Could you check a few things on this model? Use its own coordinates, in mm. A direction names the side the tool comes from. Give positions to 0.01 mm unless a question says otherwise; leave off trailing zeros. Loops run counter-clockwise (first coordinate to the right, second up) from the corner with the lowest first, then second, coordinate; pieces in that order, holes last. Notation, with made-up numbers: M 58.5,66.5 L 100.5,66.5 A11 ccw 100.5,78.5 Z; hole C 2,14.5 d7. An arc over 180 degrees is marked long. Use a Markdown table: item, result. Add a question column.
1) Suppose I cut it at D-D on z = 1.75. List the corners of the cut face in (x, y) for me, and give its area (3 significant figures).
2) Suppose I cut it at A-A on z = 6. List the corners of the cut face in (x, y) for me, and give its area (3 significant figures).
3) If I drill on line 1 along X through (y, z) = (3.45, 6); line 2 along X through (y, z) = (1.8, 6); line 3 along Z through (x, y) = (-20, 4), over which ranges is the centre line in solid material (lowest first)? Write a range as [from, to].
4) Which directions (+Z, -Z, +X, -X, +Y, -Y) give clear straight access to the entire face, cutting with the end or side of a thin tool? Please do faces 5 (the flat face through (25, 15, 1)), 6 (the flat face through (-23.487, 17.602, 0.493)), 7 (the flat face through (21.1, 5, 6)), 8 (the flat face through (-30.92, 17.91, 0.49)).
5) We'd pull the mould along X, two halves only. Please class faces 1 (the flat face through (-25, 15, 1)), 2 (the flat face through (-27.14, 11.63, 0.49)), 3 (the flat face through (30.97, 17.82, 0.49)), 4 (the flat face through (23.64, 17.69, 0.49)): +X half, -X half, draft (parallel to the pull), parting line (faces both ways), or undercut.
6) Suppose I cut it at B-B on y = 12. List the corners of the cut face in (x, z) for me, and give its area (3 significant figures).
7) Will these pins go through, and if not, where does the flat tip stop? pin 1 Ø14.5 at (x, y) = (4.5, 14) entering from +Z; pin 2 Ø3 at (x, z) = (-19.87, 6) entering from +Y; pin 3 Ø2 at (x, z) = (25, 1.5) entering from -Y.
8) Suppose I cut it at C-C on y = 17. List the corners of the cut face in (x, z) for me.
```python
from build123d import *

# Parameters (mm, degrees)
BOSS_EXTRUDE1_DEPTH = 3
BOSS_EXTRUDE2_DEPTH = 6
SKETCH4_R           = 1
CUT_EXTRUDE1_DEPTH  = 5
CUT_EXTRUDE2_DEPTH  = 2


with BuildPart() as part:
    # Sketch1 → Boss-Extrude1 (new body)
    with BuildSketch(Plane.XY):
        with BuildLine():
            Line((32.694937372, 14.834979008), (29.194937372, 20.897156835))
            Line((29.194937372, 20.897156835), (17.936607123, 14.397156835))
            ThreePointArc((17.936607123, 14.397156835), (11.5, 19.918584287), (3.5, 22.732135843))
            Line((3.5, 22.732135843), (3.5, 35.732135843))
            Line((3.5, 35.732135843), (-3.5, 35.732135843))
            Line((-3.5, 35.732135843), (-3.5, 22.732135843))
            ThreePointArc((-3.5, 22.732135843), (-11.5, 19.918584287), (-17.936607123, 14.397156835))
            Line((-17.936607123, 14.397156835), (-29.194937372, 20.897156835))
            Line((-29.194937372, 20.897156835), (-32.694937372, 14.834979008))
            Line((-32.694937372, 14.834979008), (-21.436607123, 8.334979008))
            ThreePointArc((-21.436607123, 8.334979008), (-22.605773199, 4.240167224), (-23, 0))
            Line((-23, 0), (-18, 0))
            ThreePointArc((-18, 0), (0, 18), (18, 0))
            Line((18, 0), (23, 0))
            ThreePointArc((23, 0), (22.605773199, 4.240167224), (21.436607123, 8.334979008))
            Line((21.436607123, 8.334979008), (32.694937372, 14.834979008))
        make_face()
    extrude(amount=BOSS_EXTRUDE1_DEPTH)

    # Sketch2 → Boss-Extrude2 (add)
    with BuildSketch(Plane.XY.offset(3)):
        with BuildLine():
            Line((-17.291616466, 5), (-22.449944321, 5))
            ThreePointArc((-22.449944321, 5), (-22.862072515, 2.515082566), (-23, 0))
            Line((-23, 0), (-18, 0))
            ThreePointArc((-18, 0), (-17.822024245, 2.524965704), (-17.291616466, 5))
        make_face()
        with BuildLine():
            Line((22.449944321, 5), (17.291616466, 5))
            ThreePointArc((17.291616466, 5), (17.822024245, 2.524965704), (18, 0))
            Line((18, 0), (23, 0))
            ThreePointArc((23, 0), (22.862072515, 2.515082566), (22.449944321, 5))
        make_face()
    extrude(amount=BOSS_EXTRUDE2_DEPTH)

    # Sketch4 → Cut-Extrude1 (cut)
    with BuildSketch(Plane(origin=(0, 5, 0), x_dir=(1, 0, 0), z_dir=(0, 1, 0))):
        with Locations((-19.870780393, -6)):
            Circle(SKETCH4_R)
        with Locations((19.870780393, -6)):
            Circle(SKETCH4_R)
    extrude(amount=-CUT_EXTRUDE1_DEPTH, mode=Mode.SUBTRACT)

    # Sketch5 → Cut-Extrude2 (cut)
    with BuildSketch(Plane.XY.offset(3)):
        with BuildLine():
            Line((-32.694937372, 14.834979008), (-21.436607123, 8.334979008))
            ThreePointArc((-21.436607123, 8.334979008), (-19.918584287, 11.5), (-17.936607123, 14.397156835))
            Line((-17.936607123, 14.397156835), (-29.194937372, 20.897156835))
            Line((-29.194937372, 20.897156835), (-32.694937372, 14.834979008))
        make_face()
        with BuildLine():
            ThreePointArc((-3.5, 22.732135843), (0, 23), (3.5, 22.732135843))
            Line((3.5, 22.732135843), (3.5, 35.732135843))
            Line((3.5, 35.732135843), (-3.5, 35.732135843))
            Line((-3.5, 35.732135843), (-3.5, 22.732135843))
        make_face()
        with BuildLine():
            ThreePointArc((17.936607123, 14.397156835), (19.918584287, 11.5), (21.436607123, 8.334979008))
            Line((21.436607123, 8.334979008), (32.694937372, 14.834979008))
            Line((32.694937372, 14.834979008), (29.194937372, 20.897156835))
            Line((29.194937372, 20.897156835), (17.936607123, 14.397156835))
        make_face()
    extrude(amount=-CUT_EXTRUDE2_DEPTH, mode=Mode.SUBTRACT)


solid = part.part
```
Answer block:
| question | item | result |
|---|---|---|
| 1 | outline | M -23,0 L -18,0 A18 cw 18,0 L 23,0 A23 ccw Z |
| 1 | area | 322 mm^2 |
| 2 | outline | M -23,0 L -20.87,0 L -20.87,5 L -22.45,5 A23 ccw Z; M -18.87,0 L -18,0 A18 cw -17.29,5 L -18.87,5 Z; M 17.29,5 A18 cw 18,0 L 18.87,0 L 18.87,5 Z; M 20.87,0 L 23,0 A23 ccw 22.45,5 L 20.87,5 Z |
| 2 | area | 30.5 mm^2 |
| 3 | line 1 | x = [-22.74, -20.87], [-18.87, -17.67], [17.67, 18.87], [20.87, 22.74] |
| 3 | line 2 | x = [-22.93, -20.87], [-18.87, -17.91], [17.91, 18.87], [20.87, 22.93] |
| 3 | line 3 | z = [0, 5.01], [6.99, 9] |
| 4 | face 5 | +Z, +X, +Y |
| 4 | face 6 | +Z, -Z, +Y |
| 4 | face 7 | +Z, +X, -X, +Y |
| 4 | face 8 | +Z, -Z, -X, +Y |
| 5 | face 1 | draft |
| 5 | face 2 | -X half |
| 5 | face 3 | +X half |
| 5 | face 4 | undercut |
| 6 | outline | M -27.78,0 L -13.42,0 L -13.42,3 L -19.62,3 L -19.62,1 L -27.78,1 Z; M 13.42,0 L 27.78,0 L 27.78,1 L 19.62,1 L 19.62,3 L 13.42,3 Z |
| 6 | area | 53.6 mm^2 |
| 7 | pin 1 | stops at z = 3 |
| 7 | pin 2 | stops at y = 5 |
| 7 | pin 3 | stops at y = 9.89 |
| 8 | outline | M -31.44,0 L -22.44,0 L -22.44,1 L -31.44,1 Z; M -15.49,0 L -5.92,0 L -5.92,3 L -15.49,3 Z; M 5.92,0 L 15.49,0 L 15.49,3 L 5.92,3 Z; M 22.44,0 L 31.44,0 L 31.44,1 L 22.44,1 Z |
